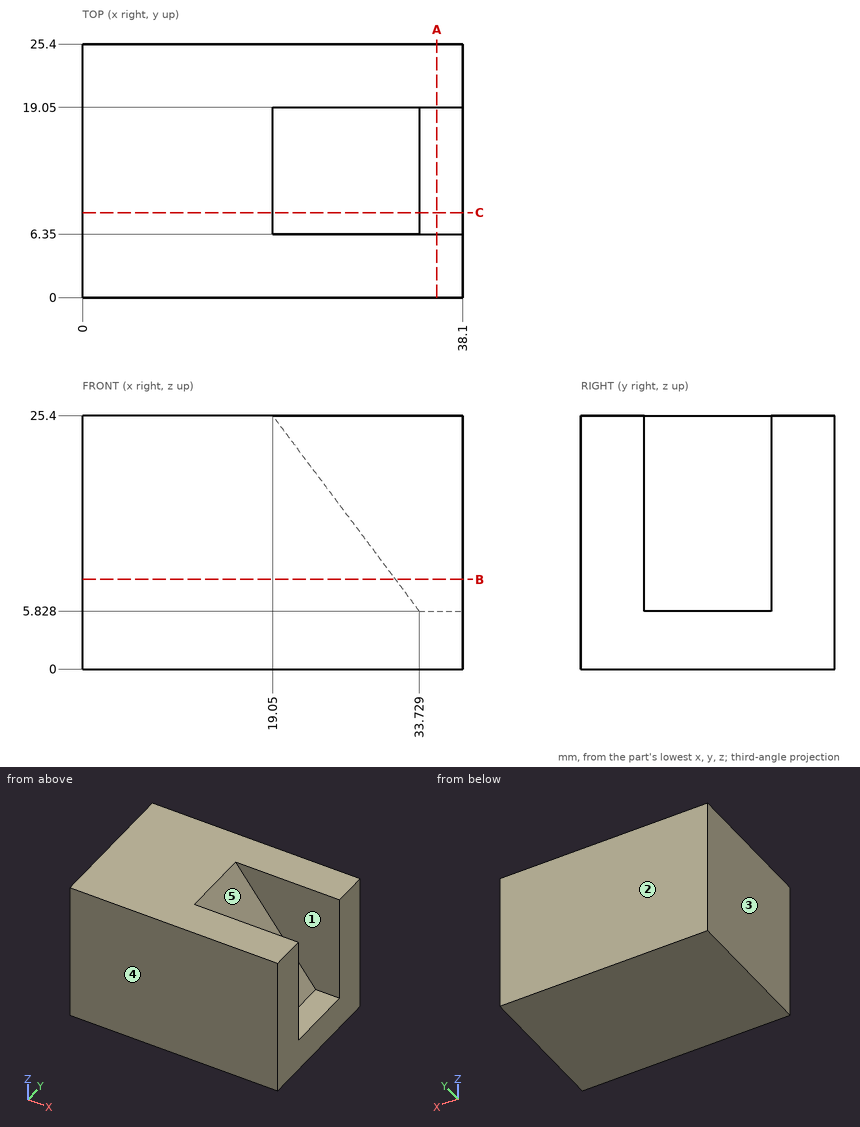
Print and shaded views of the part. All mm, measured from the part's lowest x, y and z. A direction names the side the tool comes from. Coordinates: 2 decimals unless noted, no trailing zeros. Loops run counter-clockwise (first coordinate to the right, second up) from the corner with the lowest first, then second, coordinate; pieces in that order, holes last. Notation, with made-up numbers: M 17,-15.5 L 34,-15.5 A22 cw 34,-7.5 Z; hole C 29,75 d5. An arc over 180 degrees is marked long. Use a Markdown table: item, result. Add a question column.
Q1. Cut at C-C (y = 8.5). Write the cut outline in (x, z).
Q2. Cut at B-B (z = 9). Write the cut outline in (x, y).
Q3. Mould opens along Y. For the marked faces 3, 4 and 5 say: +Y half, -Y half, draft (parallel to the pull), parting line (faces both ways), or undercut.
Q4. Which spindle directions (+Z, -Z, +X, -X, +Y, -Y) get a long thin tool onto all of the face, cutting with end or side? Do the marked faces 1 and 2. Say none if no direction does.
Q5. Cut at A-A (x = 35.5). Write the cut outline in (y, z).
Q6. Pin check, flat tip, straight feed: P1, Ø2, axis at x = 36.5, y = 11, coming from the +Z side. Stop position of the tip, or through.
Q7. Probe L1, parallel to Y at x = 33, z = 7.25; L2, parallel to Z at x = 36.5, y = 9; L3, parallel to X at y = 13.25, z = 6.25. List the from-to ranges inside material, lowest first.
Worked out:
| question | item | result |
|---|---|---|
| 1 | outline | M 0,0 L 38.1,0 L 38.1,5.83 L 33.73,5.83 L 19.05,25.4 L 0,25.4 Z |
| 2 | outline | M 0,0 L 38.1,0 L 38.1,6.35 L 31.35,6.35 L 31.35,19.05 L 38.1,19.05 L 38.1,25.4 L 0,25.4 Z |
| 3 | face 3 | draft |
| 3 | face 4 | -Y half |
| 3 | face 5 | undercut |
| 4 | face 1 | +Z, +X |
| 4 | face 2 | +Z, -Z, +X, -X, +Y |
| 5 | outline | M 0,0 L 25.4,0 L 25.4,25.4 L 19.05,25.4 L 19.05,5.83 L 6.35,5.83 L 6.35,25.4 L 0,25.4 Z |
| 6 | P1 | stops at z = 5.83 |
| 7 | L1 | y = 0 to 6.35, 19.05 to 25.4 |
| 7 | L2 | z = 0 to 5.83 |
| 7 | L3 | x = 0 to 33.41 |
